Autodesk Inventor part; units mm, degrees
ref_plane "YZ Plane" through (0, 0, 0) normal (1, 0, 0) x (0, 1, 0)
ref_plane "XZ Plane" through (0, 0, 0) normal (0, 1, 0) x (-1, 0, 0)
ref_plane "XY Plane" through (0, 0, 0) normal (0, 0, 1) x (1, 0, 0)
sketch "Sketch1" plane through (0, 0, 0) normal (0, 0, 1) x (1, 0, 0)
  circle A0 centre (0, 0) radius 1.875
  circle A1 centre (0, 0) radius 2.875
  line L0 (-2.8489, -0.3866) -> (0, -21.3815) construction
  line L1 (0, -21.3815) -> (2.8489, -0.3866) construction
  line L2 (0, -26.2328) -> (0, 7.7263)
  line L3 (-4.025, 0) -> (4.025, 0)
  arc A2 (-1.25, -12.1696) -> (1.25, -12.1696) centre (0, -12) ccw
  line L4 (-1.25, -12.1696) -> (-2.8489, -0.3866)
  line L5 (1.25, -12.1696) -> (2.8489, -0.3866)
  dimension "d0" = 3.75
  dimension "d1" = 1
  dimension "d2" = 12
  dimension "d3" = 2.5
extrude "Extrusion1" add sketch "Sketch1" against normal blind 1
extrude "Extrusion2" add sketch "Sketch1" along normal blind 2.5 contours L3 A1 L2 A0 | A0 L2 A1 L3 | A0 L3 A1 L2 | L2 A1 L3 A0
properties part number "empty"
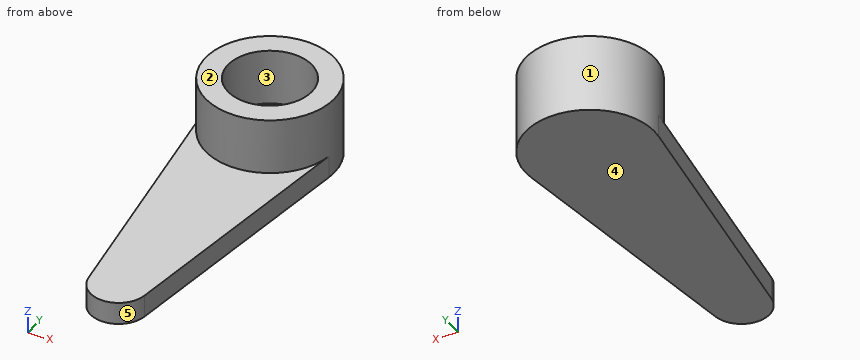
Geometry: final body of the model. Coordinates: model frame, mm. Face numbers are marked on the shaded views. A direction names the side the tool comes from. Give positions to 0.01 mm unless a question says otherwise; leave off trailing zeros. Order: outer loops, then holes, each group sorted by start corner. A loop starts at its lowest first (then second) coordinate and runs counter-clockwise, first axis right, second up. Notation, with made-up numbers: (62.25, 56.5) -> (110.25, 56.5) arc R31 cw to (110.25, 89.5) -> close; hole circle Ø9 at (11, 26). An arc over 180 degrees is marked (long way). Answer as a JSON object with one key per item and string values.
Q1. Draft query along X for the marked faces 3, 4 and 5. Return one class per face: released by +X, released by -X, zero draft, split by the parting line, or undercut.
Entries:
{"face 3": "undercut", "face 4": "zero draft", "face 5": "split by the parting line"}
Q2. Access query for the marked faces 1 and 2. Directions: +Z, -Z, +X, -X, +Y, -Y. A direction counts if a zero-diameter tool reaches every point of the face in a straight line with its end or side. Return the directions, or none.
Entries:
{"face 1": "+Z", "face 2": "+Z, +X, -X, +Y, -Y"}
Q3. Section D-D (x = 0.9). Output: boundary loops of the cut face in (y, z).
Entries:
{"outline": "(-12.88, -1) -> (2.73, -1) -> (2.73, 2.5) -> (1.64, 2.5) -> (1.64, 0) -> (-1.64, 0) -> (-1.64, 2.5) -> (-2.73, 2.5) -> (-2.73, 0) -> (-12.88, 0) -> close"}
Q4. Section B-B (x = 0). Output: boundary loops of the cut face in (y, z) (3 decimals), plus the area to 3 significant figures.
Entries:
{"outline": "(-13.261, -1) -> (2.875, -1) -> (2.875, 2.5) -> (1.875, 2.5) -> (1.875, 0) -> (-1.875, 0) -> (-1.875, 2.5) -> (-2.875, 2.5) -> (-2.875, 0) -> (-13.261, 0) -> close", "area": "21.1 mm^2"}
Q5. First-contact query: pin 1 (1.5 mm diameter, centred on y = -7.5, z = 0, fed in from +X); pin 2 (2 mm diameter, centred on x = -0.5, y = -6.5, fed in from +Z); pin 3 (1.5 mm diameter, centred on y = -2.5, z = 0.5, fed in from -X). Flat tips, straight axial feed; report the tip coordinate or a pass-through.
Entries:
{"pin 1": "stops at x = 1.99", "pin 2": "stops at z = 0", "pin 3": "stops at x = -2.64"}
Q6. Section C-C (z = 1.9). Output: boundary loops of the cut face in (x, y) (3 decimals), plus the area to 3 significant figures.
Entries:
{"outline": "circle Ø5.75 at (0, 0); hole circle Ø3.75 at (0, 0)", "area": "14.9 mm^2"}
Q7. Section A-A (y = 0). Output: boundary loops of the cut face in (x, z) (3 decimals), plus the area to 4 significant figures.
Entries:
{"outline": "(-2.875, -1) -> (2.875, -1) -> (2.875, 2.5) -> (1.875, 2.5) -> (1.875, 0) -> (-1.875, 0) -> (-1.875, 2.5) -> (-2.875, 2.5) -> close", "area": "10.75 mm^2"}
Q8. Material intervals for probe 1 along Y at (x, z) = (0, 1.4) (3 decimals); probe 2 along Z at (x, y) = (1.7, -7), sorted ascending.
Entries:
{"probe 1": "y = -2.875 to -1.875, 1.875 to 2.875", "probe 2": "z = -1 to 0"}
